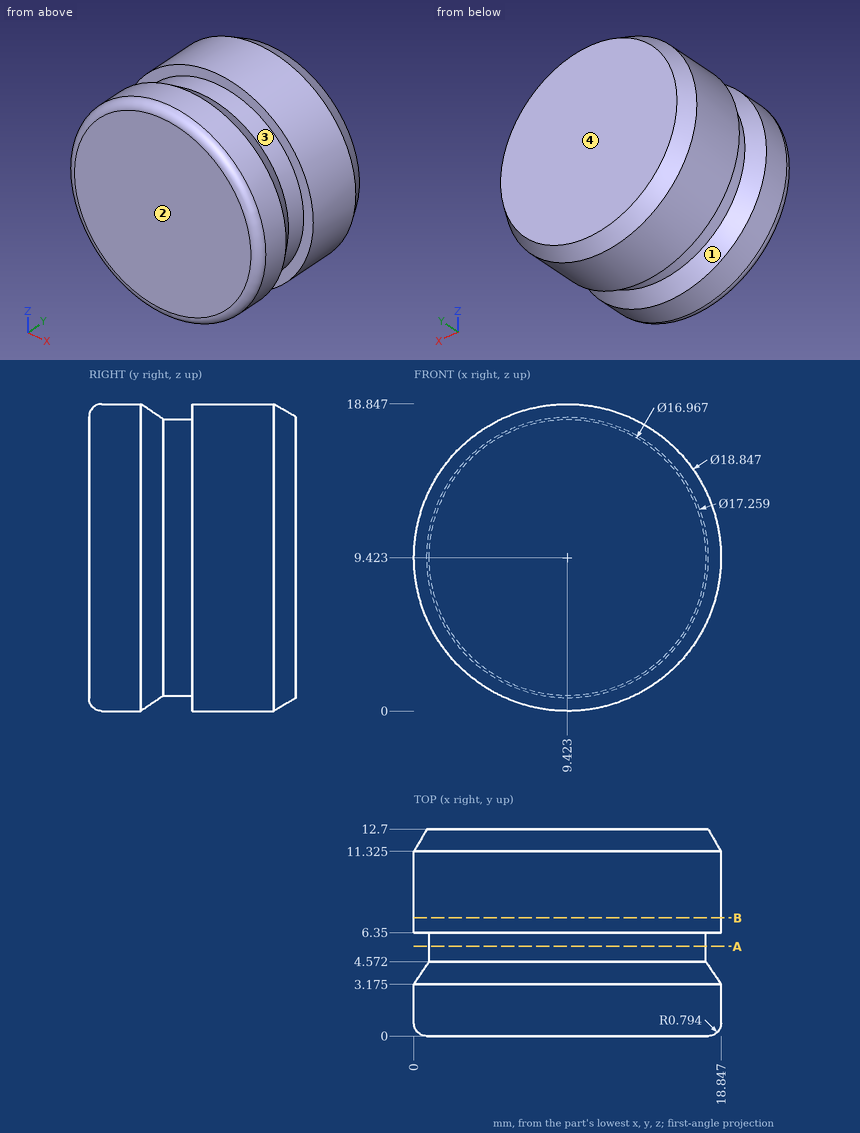
For this review, use the dimensioned drawing (mm, ordinates from the lowest corner) and the shaded views. Round coordinates to 2 decimals unless told otherwise and drop trailing zeros. Write each loop counter-clockwise with the first axis right and the second up, starting at its lowest first coordinate (ties: lowest second). Pieces come first, ordered by that corner, then holes. Notation, with made-up numbers: M -2.75,43.25 L 26.25,43.25 A30 cw 26.25,76.25 Z; hole C 7,-21.5 d7. An arc over 180 degrees is marked long. Write item = value, one per line. Start each with the question number.
(1) We need section A-A (y = 5.5). Give the boundary of the cut face in (x, z), then the cut area to 3 significant figures.
(2) For line 1 along Z through (x, y) = (1, 3.5) (1 decimal); line 2 along Z through (x, y) = (16.25, 7.75) (1 decimal); line 3 along X through (y, z) = (10.5, 5.5) (1 decimal), list the stretches that pass through material, from the lowest coordinate up.
(3) We need section B-B (y = 7.25). Give the boundary of the cut face in (x, z), then the cut area to 3 significant figures.
(4) Clearance check with flat-ended pins moving along their axes: pin 1 Ø1 at (y, z) = (11, 6.5) entering from +X; pin 2 Ø1 at (y, z) = (8.5, 6) entering from -X (1 decimal); pin 3 Ø6 at (x, y) = (5.5, 6.5) entering from -Z (1 decimal). State where each tip first meets the part, or that it passes through.
(5) The part is to be moulded in two halves that separate along Y. For the marked faces 1, 2, 3 and 4, say which applies: +Y half, -Y half, draft (parallel to the pull), parting line (faces both ways), or undercut.
Results found:
q1.outline = C 9.42,9.42 d16.97
q1.area = 226 mm²
q2.line_1 = 5.7 to 13.1
q2.line_2 = 2.9 to 15.9
q2.line_3 = 0.9 to 18
q3.outline = C 9.42,9.42 d18.85
q3.area = 279 mm²
q4.pin_1 = 18.53
q4.pin_2 = 0.5
q4.pin_3 = 0
q5.face_1 = undercut
q5.face_2 = -Y half
q5.face_3 = undercut
q5.face_4 = +Y half
